Read the model definition and answer for the solid it produces. Units are mm, in the model's axes. Face numbers are marked on the shaded views. A direction names the side the tool comes from. Give positions to 0.01 mm unless a question says otherwise; leave off trailing zeros. Order: outer loops, then holes, each group sorted by start corner. A loop starts at its lowest first (then second) coordinate and runs counter-clockwise, first axis right, second up. Notation, with made-up numbers: (74.25, 89) - (122.25, 89) arc R19 ccw to (122.25, 98) - close; hole circle Ø2 at (77, -36.75). An arc over 180 degrees is marked (long way). Write each question's results on one line, items separated by ' | '. Start each with the question number.
Q1. Find the intervals of material crossed by line 1 along Y through (x, z) = (2.2, -0.35); line 2 along X through (y, z) = (-1.25, -0.55); line 3 along X through (y, z) = (-2.25, -0.4), in increasing order. Write a range as from..to.
Q2. Find section C-C on z = 0. Give the vertices of the cut face in (x, y) (3 decimals).
Q3. Find section B-B on x = 0. Give the vertices of the cut face in (y, z) (3 decimals).
Q4. Find section A-A on y = -1.75. Give the vertices of the cut face in (x, z).
Q5. A tool of negligible diameter and unlimited length cuts with its end or side. For the marked faces 1, 2 and 3, from which of +Z, -Z, +X, -X, +Y, -Y can it reach the whole face along a straight path? Write none if from no direction.
Q6. Find section D-D on z = 0.75. Give the vertices of the cut face in (x, y) (3 decimals), and give its area (3 significant figures).
Q7. Flat-ended cylindrical pins translate along their axes: P1, Ø1.5, axis at x = 0, y = -1, coming from the +Z side; P2, Ø1, axis at x = 0, y = -3, coming from the -Z side; P3, Ø1, axis at x = -1.5, y = -6, coming from the -Z side. Find the tip coordinate at first contact, or state that the pin passes through.
from build123d import *

# Parameters (mm, degrees)
SKETCH_1_R      = 2.5
EXTRUDE_1_DEPTH = 0.5
SKETCH_4_R      = 2
EXTRUDE_2_DEPTH = 7
SKETCH_5_W      = 0.3
SKETCH_5_H      = 0.29255476
SKETCH_5_W_2    = 0.29255476
SKETCH_5_H_2    = 0.3
EXTRUDE_3_DEPTH = 2


with BuildPart() as part:
    # 草图1 → 凸台-拉伸1 (new body)
    with BuildSketch(Plane(origin=(0, 0, 0), x_dir=(1, 0, 0), z_dir=(0, 1, 0))):
        with Locations(Location((0, 0, 0), (0, 0, 270))):
            Circle(SKETCH_1_R)
    extrude(amount=EXTRUDE_1_DEPTH)

    # 草图2 → 旋转4 (revolve)
    with BuildSketch(Plane.XY):
        with BuildLine():
            Line((2.5, 0), (0, 0))
            Line((0, 0), (0, 1.25))
            ThreePointArc((0, 1.25), (1.397542486, 0.920084972), (2.5, 0))
        make_face()
    revolve(axis=Axis((0, 3.671150215, 0), (0, -1, 0)))

    # 草图4 → 凸台-拉伸2 (add)
    with BuildSketch(Plane.XZ):
        with Locations(Location((0, 0, 0), (0, 0, 90))):
            Circle(SKETCH_4_R)
    extrude(amount=EXTRUDE_2_DEPTH)

    # 草图5 → 凸台-拉伸3 (add)
    with BuildSketch(Plane.XZ):
        with Locations((0, 2.05372262)):
            Rectangle(SKETCH_5_W, SKETCH_5_H)
        with Locations((-2.05372262, 0)):
            Rectangle(SKETCH_5_W_2, SKETCH_5_H_2)
        with Locations((2.05372262, 0)):
            Rectangle(SKETCH_5_W_2, SKETCH_5_H_2)
        with Locations((0, -2.05372262)):
            Rectangle(SKETCH_5_W, SKETCH_5_H)
    extrude(amount=EXTRUDE_3_DEPTH)


solid = part.part
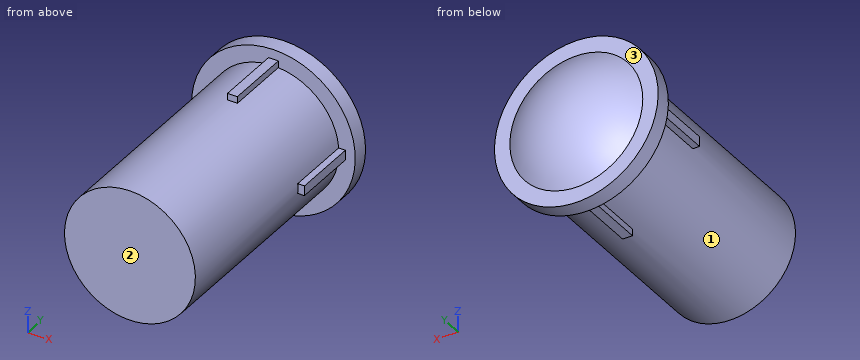
Working result:
1) line 1: 0..0.5 | line 2: -1.92..1.92 | line 3: -1.96..1.96
2) outline: (-2.5, 0) - (-2.2, 0) - (-2.2, -2) - (-2, -2) - (-2, -7) - (2, -7) - (2, -2) - (2.2, -2) - (2.2, 0) - (2.5, 0) - (2.5, 0.5) - (2.031, 0.5) arc R3.125 ccw to (-2.031, 0.5) - (-2.5, 0.5) - close
3) outline: (-7, -2) - (-2, -2) - (-2, -2.2) - (0, -2.2) - (0, -2.5) - (0.5, -2.5) - (0.5, -2.031) arc R3.125 ccw to (0.5, 2.031) - (0.5, 2.5) - (0, 2.5) - (0, 2.2) - (-2, 2.2) - (-2, 2) - (-7, 2) - close
4) outline: (-2.2, -0.15) - (-1.99, -0.15) arc R2 ccw to (-0.15, -1.99) - (-0.15, -2.2) - (0.15, -2.2) - (0.15, -1.99) arc R2 ccw to (1.99, -0.15) - (2.2, -0.15) - (2.2, 0.15) - (1.99, 0.15) arc R2 ccw to (0.15, 1.99) - (0.15, 2.2) - (-0.15, 2.2) - (-0.15, 1.99) arc R2 ccw to (-1.99, 0.15) - (-2.2, 0.15) - close
5) face 1: -Y | face 2: +Z, -Z, +X, -X, -Y | face 3: +Y
6) outline: (-2.385, 0) - (-1.854, 0) - (-1.854, -7) - (1.854, -7) - (1.854, 0) - (2.385, 0) - (2.385, 0.5) - (1.887, 0.5) arc R3.034 ccw to (-1.887, 0.5) - (-2.385, 0.5) - close | area: 30.0 mm²
7) P1: z = 2.2 | P2: z = -2 | P3: z = -1.73
